The listing builds one solid part. Answer for the finished solid, in the listing's coordinates (mm). A direction names the side the tool comes from. Give positions to 0.01 mm unless a question says otherwise; leave off trailing zeros. Write each loop counter-clockwise with the first axis right and the second up, starting at its lowest first coordinate (ties: lowest second). Pieces come first, ordered by that corner, then holes. Notation, with made-up numbers: (86, 33.5) - (100, 33.5) arc R24 cw to (100, 66.5) - close; hole circle Ø5 at (-9.5, 75). An arc over 180 degrees is marked (long way). One line per question, with ' | ' between items. Start each with the question number.
1. A cutting plane is placed at C-C (y = 21). Determine the outline of the cut face in (x, z).
2. A cutting plane is placed at B-B (x = 17). Determine the outline of the cut face in (y, z), then the cut area to 4 significant figures.
3. Find the intervals of material crossed by L1, parallel to Y at x = 12, z = 81; L2, parallel to X at y = 34.5, z = 167; L3, parallel to X at y = 45, z = 566, in increasing order. Write a range as from..to.
4. For faces 1 (the face through (4.5, 25, 296)), 2 (the face through (4, 23, 600)), determine the directions among +Z, -Z, +X, -X, +Y, -Y from which every point of the face is accessible in a straight line to the end or side of a thin tool.
5. A cutting plane is placed at A-A (z = 232). Determine the outline of the cut face in (x, y) (3 decimals).
6. Given P1, Ø2, axis at y = 35, z = 320.5, coming from the +X side; P2, Ø23, axis at y = 26, z = 281, coming from the +X side, each flat-ended and moving along its own axis, determine where each tip first touches the part or whether it passes through.
7. The mould has two halves that part along Y. Classify faces 3 (the face through (22.65, 43.41, 295.8)), 4 (the face through (22.35, 6.61, 295.8)), 5 (the face through (19, 0, 296)), 6 (the face through (4, 23, 0)): +Y half, -Y half, draft (parallel to the pull), parting line (faces both ways), or undercut.
```python
from build123d import *

# Parameters (mm, degrees)
EXTRUDE_1_DEPTH = 600


with BuildPart() as part:
    # 草图1 → 拉伸1 (new body)
    with BuildSketch(Plane.XY):
        with BuildLine():
            Line((4.5, 35.525), (4.5, 14.475))
            ThreePointArc((4.5, 14.475), (6.550252532, 9.525252532), (11.5, 7.475))
            Line((11.5, 7.475), (33.5, 5.725))
            ThreePointArc((33.5, 5.725), (35.974873734, 4.699873734), (37, 2.225))
            Line((37, 2.225), (37, 0))
            Line((37, 0), (0, 0))
            Line((0, 0), (0, 50))
            Line((0, 50), (37, 50))
            Line((37, 50), (37, 47.775))
            ThreePointArc((37, 47.775), (35.974873734, 45.300126266), (33.5, 44.275))
            Line((33.5, 44.275), (11.5, 42.525))
            ThreePointArc((11.5, 42.525), (6.550252532, 40.474747468), (4.5, 35.525))
        make_face()
        with BuildLine():
            Line((0, 50), (0, 25))
            Line((0, 25), (4.5, 25))
            Line((4.5, 25), (4.5, 35.525))
            ThreePointArc((4.5, 35.525), (6.550252532, 40.474747468), (11.5, 42.525))
            Line((11.5, 42.525), (33.5, 44.275))
            ThreePointArc((33.5, 44.275), (35.974873734, 45.300126266), (37, 47.775))
            Line((37, 47.775), (37, 50))
            Line((37, 50), (0, 50))
        make_face()
    extrude(amount=EXTRUDE_1_DEPTH)


solid = part.part
```
Determined:
1) outline: (0, 0) - (4.5, 0) - (4.5, 600) - (0, 600) - close
2) outline: (0, 0) - (7.04, 0) - (7.04, 600) - (0, 600) - close; (42.96, 0) - (50, 0) - (50, 600) - (42.96, 600) - close | area: 8,445 mm2
3) L1: 0..7.44, 42.56..50 | L2: 0..4.5 | L3: 0..35.63
4) face 1: +Z, -Z, +X | face 2: +Z, +X, -X, +Y, -Y
5) outline: (0, 0) - (37, 0) - (37, 2.225) arc R3.5 ccw to (33.5, 5.725) - (11.5, 7.475) arc R7 cw to (4.5, 14.475) - (4.5, 35.525) arc R7 cw to (11.5, 42.525) - (33.5, 44.275) arc R3.5 ccw to (37, 47.775) - (37, 50) - (0, 50) - close
6) P1: x = 4.52 | P2: x = 4.78
7) face 3: undercut | face 4: undercut | face 5: -Y half | face 6: draft
